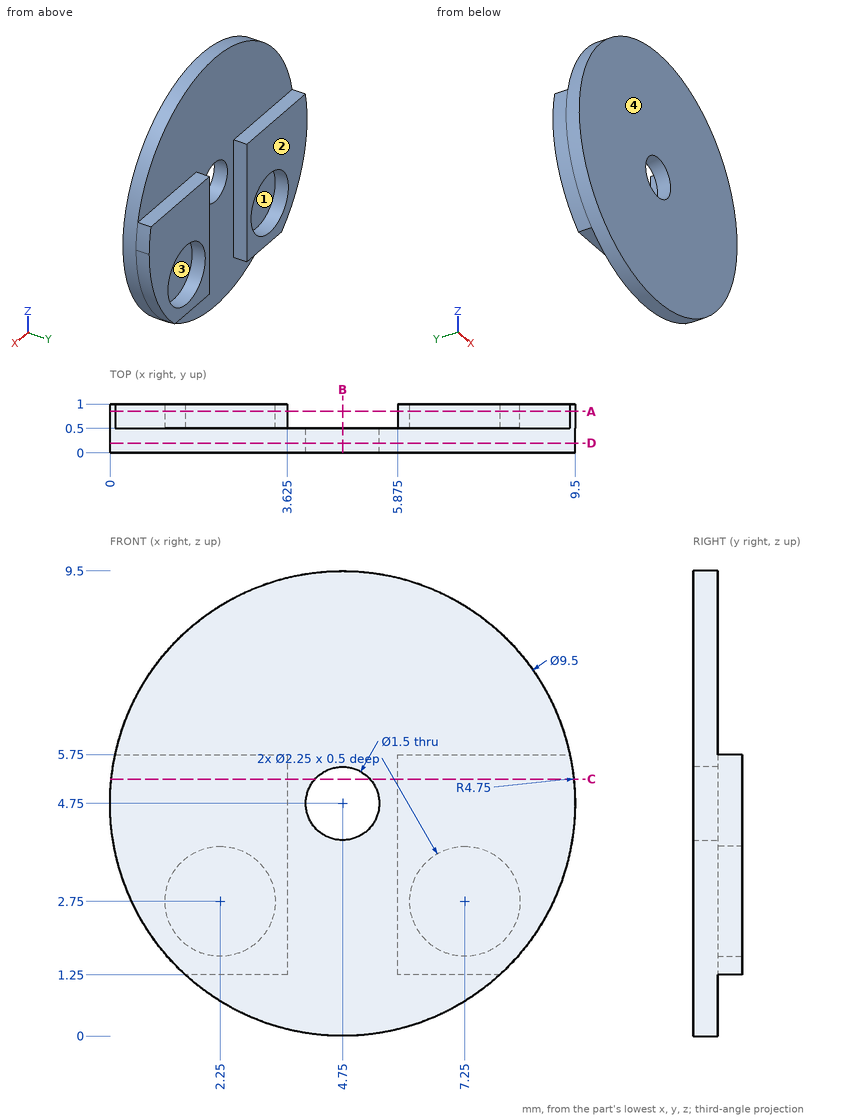
Geometry: see drawing. Coordinates: mm, zero at the bounding-box minimum. A direction names the side the tool comes from. Give positions to 0.01 mm unless a question says otherwise; leave off trailing zeros. Write each loop counter-clockwise with the first axis right and the second up, starting at its lowest first coordinate (ties: lowest second). Pieces come first, ordered by that corner, then holes. Notation, with made-up numbers: M 2,-6.75 L 60,-6.75 A15 cw 60,20.25 Z; hole C 86.25,-14.5 d6. An arc over 180 degrees is marked long. Answer in a Markdown table with one row per item. Add a question column.
(1) Mould query, pull axis Y, two halves, no side actions, for the marked faces 3 and 4. Classes: +Y half, -Y half, draft (parallel to the pull), parting line (faces both ways), or undercut.
(2) Section C-C on z = 5.25. Return loops of the section in (x, y) (3 decimals).
(3) Section A-A on y = 0.85. Return loops of the section in (x, z) (3 decimals).
(4) First-contact query: pin 1 (0.9 mm diameter, centred on x = 4.75, z = 4.75, fed in from -Y); pin 2 (2 mm diameter, centred on x = 4.5, z = 7, fed in from +Y); pin 3 (0.6 mm diameter, centred on x = 2.5, y = 0.5, fed in from -Z). Flat tips, straight axial feed; report the tip coordinate or a pass-through.
(5) Ray query, line 1 (X direction, y = 0.85, z = 2.75) (3 decimals); line 2 (X direction, y = 0.6, z = 1.75) (3 decimals); line 3 (Y direction, x = 6.75, z = 2.5). Return the intervals inside material, ascending.
(6) Section B-B on x = 4.75. Return loops of the section in (y, z), and give its area (3 significant figures).
(7) Section D-D on y = 0.2. Return loops of the section in (x, z).
(8) Reachability of the marked faces 1 and 2 from +Z, -Z, +X, -X, +Y, -Y: full face, straight path, thin tool, end or side. Return the list, or none.
Result set:
| question | item | result |
|---|---|---|
| 1 | face 3 | +Y half |
| 1 | face 4 | -Y half |
| 2 | outline | M 0.026,0 L 4.191,0 L 4.191,0.5 L 3.625,0.5 L 3.625,1 L 0.026,1 Z; M 5.309,0 L 9.474,0 L 9.474,1 L 5.875,1 L 5.875,0.5 L 5.309,0.5 Z |
| 3 | outline | M 0.106,5.75 A4.75 ccw 1.539,1.25 L 3.625,1.25 L 3.625,5.75 Z; M 5.875,1.25 L 7.961,1.25 A4.75 ccw 9.394,5.75 L 5.875,5.75 Z; hole C 2.25,2.75 d2.25; hole C 7.25,2.75 d2.25 |
| 4 | pin 1 | passes through |
| 4 | pin 2 | stops at y = 0.5 |
| 4 | pin 3 | stops at z = 0.42 |
| 5 | line 1 | x = 0.442 to 1.125, 3.375 to 3.625, 5.875 to 6.125, 8.375 to 9.058 |
| 5 | line 2 | x = 1.067 to 1.735, 2.765 to 3.625, 5.875 to 6.735, 7.765 to 8.433 |
| 5 | line 3 | y = 0 to 0.5 |
| 6 | outline | M 0,0 L 0.5,0 L 0.5,4 L 0,4 Z; M 0,5.5 L 0.5,5.5 L 0.5,9.5 L 0,9.5 Z |
| 6 | area | 4.00 mm^2 |
| 7 | outline | C 4.75,4.75 d9.5; hole C 4.75,4.75 d1.5 |
| 8 | face 1 | +Y |
| 8 | face 2 | +Z, -Z, +X, -X, +Y |
